Input: dimensioned drawing with shaded views. Units: mm. Origin: part minimum x, y, z. A direction names the side the tool comes from. Give positions to 0.01 mm unless a question says otherwise; leave off trailing zeros. Write each loop counter-clockwise with the first axis right and the second up, starting at its lowest first coordinate (ties: lowest second). Pieces come first, ordered by that corner, then holes.
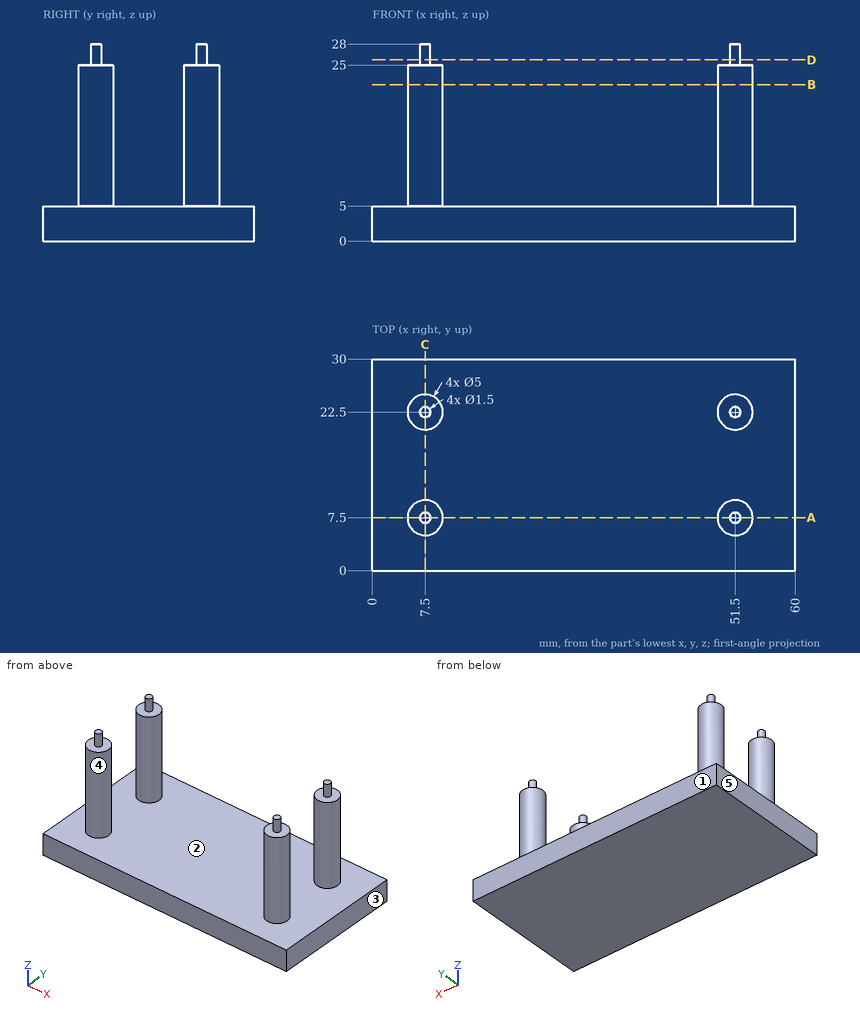
Item 1: Line query: L1, parallel to Z at x = 30, y = 28; L2, parallel to Z at x = 50.5, y = 23.5; L3, parallel to Y at x = 52.5, z = 14. Output: solid intervals per line, ascending.
Found:
L1: z = 0 to 5
L2: z = 0 to 25
L3: y = 5.21 to 9.79, 20.21 to 24.79
Item 2: Reachability of the marked faces 1 and 2 from +Z, -Z, +X, -X, +Y, -Y: full face, straight path, thin tool, end or side. Return the list, or none.
Found:
face 1: +Z, -Z, +X, -X, +Y
face 2: +Z
Item 3: Section D-D, the plane z = 25.75. Return the cut outline in (x, y), plus the area to 3 significant figures.
Found:
outline: circle Ø1.5 at (7.5, 7.5); circle Ø1.5 at (7.5, 22.5); circle Ø1.5 at (51.5, 7.5); circle Ø1.5 at (51.5, 22.5)
area: 7.07 mm2
Item 4: Pin query (flat end, axial travel): pin 1 Ø5 at (y, z) = (6, 8.5) entering from +X; pin 2 Ø3 at (y, z) = (23.5, 8.5) entering from -X; pin 3 Ø3 at (y, z) = (24.5, 15.5) entering from -X. Return the tip coordinate at first contact, or that it passes through.
Found:
pin 1: stops at x = 54
pin 2: stops at x = 5
pin 3: stops at x = 5.05
Item 5: Section A-A, the plane y = 7.5. Return the cut outline in (x, z), plus the area to 3 significant figures.
Found:
outline: (0, 0) - (60, 0) - (60, 5) - (54, 5) - (54, 25) - (52.25, 25) - (52.25, 28) - (50.75, 28) - (50.75, 25) - (49, 25) - (49, 5) - (10, 5) - (10, 25) - (8.25, 25) - (8.25, 28) - (6.75, 28) - (6.75, 25) - (5, 25) - (5, 5) - (0, 5) - close
area: 509 mm2
Item 6: Section B-B, the plane z = 22.25. Return the cut outline in (x, y).
Found:
outline: circle Ø5 at (7.5, 7.5); circle Ø5 at (7.5, 22.5); circle Ø5 at (51.5, 7.5); circle Ø5 at (51.5, 22.5)
Item 7: Pull-direction query (X, two-part tool) for the marked faces 3, 4 and 5; classes: +X half, -X half, draft (parallel to the pull), parting line (faces both ways), or undercut.
Found:
face 3: +X half
face 4: undercut
face 5: -X half
Item 8: Section C-C, the plane x = 7.5. Return the cut outline in (y, z).
Found:
outline: (0, 0) - (30, 0) - (30, 5) - (25, 5) - (25, 25) - (23.25, 25) - (23.25, 28) - (21.75, 28) - (21.75, 25) - (20, 25) - (20, 5) - (10, 5) - (10, 25) - (8.25, 25) - (8.25, 28) - (6.75, 28) - (6.75, 25) - (5, 25) - (5, 5) - (0, 5) - close
